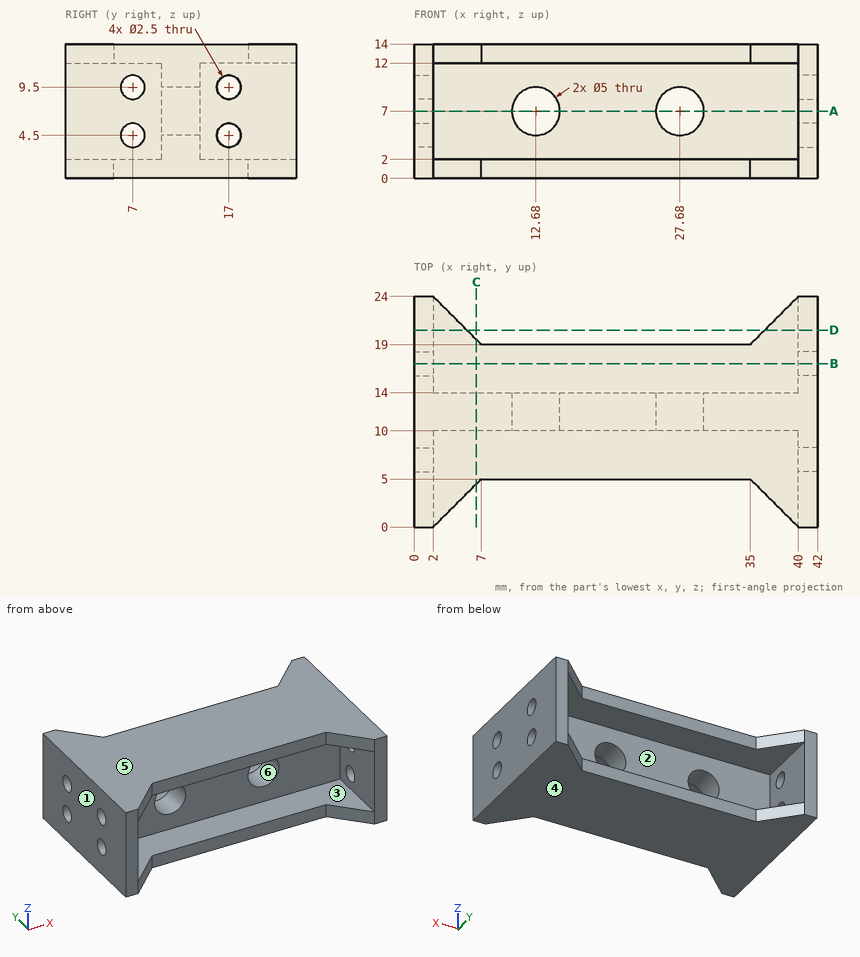
Job drawing, mm, ordinate dimensions from the low corner. One solid piece. A direction names the side the tool comes from. Give positions to 0.01 mm unless a question says otherwise; leave off trailing zeros. Loops run counter-clockwise (first coordinate to the right, second up) from the corner with the lowest first, then second, coordinate; pieces in that order, holes last. Notation, with made-up numbers: M -6,67 L 31,67 A19 cw 31,99 Z; hole C 71.25,-16.5 d7. An arc over 180 degrees is marked long. Put each result on its own line as item: value. Start each with the question number.
1) Pull direction Z, two halves, no side cores. Call the marked faces 4, 5 and 6: +Z half, -Z half, draft (parallel to the pull), parting line (faces both ways), or undercut.
2) Saw through at D-D (y = 20.5). List the corners of the cut face in (x, z).
3) 3-axis set-ups, long thin cutter, end or side, ignore diameter. For the marked faces 1, 2 and 3: which of +Z, -Z, +X, -X, +Y, -Y reach the whole face in a straight line?
4) Saw through at A-A (z = 7). List the corners of the cut face in (x, y).
5) Flat gauge pins, fed straight in: pin 1 (6 mm diameter, centred on x = 26, z = 8, fed in from +Y); pin 2 (1.6 mm diameter, centred on x = 18, z = 1, fed in from -Y); pin 3 (8 mm diameter, centred on x = 12.68, z = 7, fed in from -Y). Where does each tip first touch, or does it go through?
6) Probe probe 1 along Y at (x, z) = (1.2, 4.5); probe 2 along Z at (x, y) = (21, 16); probe 3 along X at (y, z) = (19, 7.75). List the from-to ranges inside material, lowest first.
7) Saw through at C-C (x = 6.5). List the corners of the cut face in (y, z), then the cut area to 4 significant figures.
8) Saw through at B-B (y = 17). List the corners of the cut face in (x, z).
Numbers:
1. face 4: -Z half
1. face 5: +Z half
1. face 6: undercut
2. outline: M 0,0 L 5.5,0 L 5.5,2 L 2,2 L 2,12 L 5.5,12 L 5.5,14 L 0,14 Z; M 36.5,0 L 42,0 L 42,14 L 36.5,14 L 36.5,12 L 40,12 L 40,2 L 36.5,2 Z
3. face 1: +Z, -Z, -X, +Y, -Y
3. face 2: +Y
3. face 3: -Y
4. outline: M 0,0 L 2,0 L 2,10 L 10.18,10 L 10.18,14 L 2,14 L 2,24 L 0,24 Z; M 15.18,10 L 25.18,10 L 25.18,14 L 15.18,14 Z; M 30.18,10 L 40,10 L 40,0 L 42,0 L 42,24 L 40,24 L 40,14 L 30.18,14 Z
5. pin 1: y = 14
5. pin 2: y = 5
5. pin 3: y = 10
6. probe 1: 0 to 5.75, 8.25 to 15.75, 18.25 to 24
6. probe 2: 0 to 2, 12 to 14
6. probe 3: 0 to 2, 40 to 42
7. outline: M 4.5,0 L 19.5,0 L 19.5,2 L 14,2 L 14,12 L 19.5,12 L 19.5,14 L 4.5,14 L 4.5,12 L 10,12 L 10,2 L 4.5,2 Z
7. area: 100.0 mm^2
8. outline: M 0,0 L 42,0 L 42,3.25 L 40,3.25 L 40,2 L 2,2 L 2,3.25 L 0,3.25 Z; M 0,5.75 L 2,5.75 L 2,8.25 L 0,8.25 Z; M 0,10.75 L 2,10.75 L 2,12 L 40,12 L 40,10.75 L 42,10.75 L 42,14 L 0,14 Z; M 40,5.75 L 42,5.75 L 42,8.25 L 40,8.25 Z
